Design review of the part built by this model. Coordinates are the model's own, in mm. A direction names the side the tool comes from. Coordinates: 2 decimals unless noted, no trailing zeros. Loops run counter-clockwise (first coordinate to the right, second up) from the corner with the lowest first, then second, coordinate; pieces in that order, holes last. Notation, with made-up numbers: (-34, 29) - (14, 29) arc R24 cw to (14, 40) - close; hole circle Ø1 at (-33, 20.25). An arc over 180 degrees is marked (long way). Return JSON: item names as keys, results as strings. Group by question number.
from build123d import *

# Parameters (mm, degrees)
SKETCH_W        = 48
SKETCH_H        = 39
PAD_DEPTH       = 50
SKETCH001_R     = 10.5
POCKET_DEPTH    = 51
SKETCH002_R     = 12.5
POCKET001_DEPTH = 5
SKETCH003_R     = 12.5
POCKET002_DEPTH = 5
POCKET003_DEPTH = 51
SKETCH005_R     = 2.5
POCKET004_DEPTH = 20


with BuildPart() as part:
    # Sketch → Pad (new body)
    with BuildSketch(Plane.XY):
        with Locations((24, 19.5)):
            Rectangle(SKETCH_W, SKETCH_H)
    extrude(amount=PAD_DEPTH)

    # Sketch001 → Pocket (cut)
    with BuildSketch(Plane.XY.offset(50)):
        with Locations((24, 16)):
            Circle(SKETCH001_R)
    extrude(amount=-POCKET_DEPTH, mode=Mode.SUBTRACT)

    # Sketch002 → Pocket001 (cut)
    with BuildSketch(Plane.XY.offset(50)):
        with Locations((24, 16)):
            Circle(SKETCH002_R)
    extrude(amount=-POCKET001_DEPTH, mode=Mode.SUBTRACT)

    # Sketch003 → Pocket002 (cut)
    with BuildSketch(Plane(origin=(0, 0, 0), x_dir=(1, 0, 0), z_dir=(0, 0, -1))):
        with Locations((24, -16)):
            Circle(SKETCH003_R)
    extrude(amount=-POCKET002_DEPTH, mode=Mode.SUBTRACT)

    # Sketch004 → Pocket003 (cut)
    with BuildSketch(Plane.XY.offset(50)):
        Polygon((14, 0), (24, 16), (34, 0), align=None)
    extrude(amount=-POCKET003_DEPTH, mode=Mode.SUBTRACT)

    # Sketch005 → Pocket004 (cut)
    with BuildSketch(Plane(origin=(0, 39, 0), x_dir=(-1, 0, 0), z_dir=(0, 1, 0))):
        with Locations((-41.5, 42.5)):
            Circle(SKETCH005_R)
        with Locations((-6.5, 42.5)):
            Circle(SKETCH005_R)
        with Locations((-41.5, 7.5)):
            Circle(SKETCH005_R)
        with Locations((-6.5, 7.5)):
            Circle(SKETCH005_R)
    extrude(amount=-POCKET004_DEPTH, mode=Mode.SUBTRACT)


solid = part.part
Item 1: Add section A-A (y = 16). State the section outline as (x, z) points.
Item 2: Add section B-B (x = 6.5). State the section outline as (y, z) points.
Item 3: For P1, Ø2.5, axis at x = 41.5, z = 8, coming from the +Y side; P2, Ø22.5, axis at x = 24, y = 16, coming from the +Z side, all flat-tipped, find the tip position at first contact; note any pin that passes through.
Item 4: For faces 4 (the face through (42, 19, 8)), 5 (the face through (21.2, 26.4, 45)), 6 (the face through (31.75, 3.6, 25.35)), list the 3-axis set-ups (+Z, -Z, +X, -X, +Y, -Y) from which the entire face can be reached by the end or side of a thin tool; tool diameter is ignored.
Item 5: Add section D-D (y = 30.5). State the section outline as (x, z) points, then the cut area to 3 significant figures.
Item 6: Add section C-C (z = 21). State the section outline as (x, y) points, then the cut area to 3 significant figures.
Item 7: To check wall thickness, follow line 1 (Z direction, x = 41.5, y = 32.75); line 2 (Z direction, x = 42, y = 21.5); line 3 (X direction, y = 16, z = 23). State the ranges of each line that lie inside material, in increasing order. Write a range as from..to.
Item 8: Draft analysis for pull direction Z (two halves, no side actions). For faces 1 (the face through (21.2, 26.3, 5)), 2 (the face through (7, 19, 8)), 3 (the face through (0, 19, 25)), state which applies: pulls with the +Z half, pulls with the -Z half, needs draft (parallel to the pull), parting line crosses it, or undercut.
Answers below:
{
 "1": {"outline": "(0, 0) - (11.5, 0) - (11.5, 5) - (13.5, 5) - (13.5, 45) - (11.5, 45) - (11.5, 50) - (0, 50) - close; (34.5, 5) - (36.5, 5) - (36.5, 0) - (48, 0) - (48, 50) - (36.5, 50) - (36.5, 45) - (34.5, 45) - close"},
 "2": {"outline": "(0, 0) - (39, 0) - (39, 5) - (19, 5) - (19, 10) - (39, 10) - (39, 40) - (19, 40) - (19, 45) - (39, 45) - (39, 50) - (0, 50) - close"},
 "3": {"P1": "stops at y = 19", "P2": "stops at z = 45"},
 "4": {"face 4": "+Y", "face 5": "+Z", "face 6": "+Z, -Z, -Y"},
 "5": {"outline": "(0, 0) - (48, 0) - (48, 50) - (0, 50) - close; hole circle Ø5 at (6.5, 7.5); hole circle Ø5 at (6.5, 42.5); hole circle Ø5 at (41.5, 7.5); hole circle Ø5 at (41.5, 42.5)", "area": "2,320 mm^2"},
 "6": {"outline": "(0, 0) - (14, 0) - (18.44, 7.1) arc R10.5 cw (long way) to (29.56, 7.1) - (34, 0) - (48, 0) - (48, 39) - (0, 39) - close", "area": "1,430 mm^2"},
 "7": {"line 1": "z = 0..5, 10..40, 45..50", "line 2": "z = 0..5.05, 9.95..40.05, 44.95..50", "line 3": "x = 0..13.5, 34.5..48"},
 "8": {"face 1": "pulls with the -Z half", "face 2": "undercut", "face 3": "needs draft"}
}
